from build123d import *

# Parameters (mm, degrees)
SKETCH2_R                    = 1.5875
MAINPLATE_DEPTH              = 8.89
SKETCH3_R                    = 3.4925
CASTERWHEEL_MOUNTHOLES_DEPTH = 3.048
SKETCH4_R                    = 2.159
ARDUINO_MOUNTHOLES_DEPTH     = 6.35
SKETCH5_R                    = 2.159
PDB_16A_MOUNTINGHOLES_DEPTH  = 6.35
SKETCH6_R                    = 2.232248555
PDB_15A_MOUNTINGHOLES_DEPTH  = 6.35
SKETCH7_R                    = 2.159
DRV8871_MOUNTINGHOLES_DEPTH  = 6.35
DRV8871_MOUNTPATTERN_COUNT   = 4
DRV8871_MOUNTPATTERN_PITCH   = 24.13
SKETCH8_R                    = 1.397
BOSS_EXTRUDE1_DEPTH          = 8.89
FILLET1_R                    = 2.54
FILLET2_R                    = 2.54


with BuildPart() as part:
    # Sketch2 → MainPlate (new body)
    with BuildSketch(Plane(origin=(0, 0, 0), x_dir=(1, 0, 0), z_dir=(0, 1, 0))):
        Polygon((-69.85, 0), (-69.85, 82.55), (69.85, 82.55), (69.85, 0), (69.85, -101.6), (-69.85, -101.6), align=None)
        with Locations(Location((30.1625, 19.05, 0), (0, 0, 270))):
            Circle(SKETCH2_R, mode=Mode.SUBTRACT)
        with Locations(Location((30.1625, -19.05, 0), (0, 0, 270))):
            Circle(SKETCH2_R, mode=Mode.SUBTRACT)
        with Locations(Location((-30.1625, -19.05, 0), (0, 0, 270))):
            Circle(SKETCH2_R, mode=Mode.SUBTRACT)
        with Locations(Location((-30.1625, 19.05, 0), (0, 0, 270))):
            Circle(SKETCH2_R, mode=Mode.SUBTRACT)
    extrude(amount=MAINPLATE_DEPTH)

    # Sketch3 → CasterWheel_MountHoles (cut)
    with BuildSketch(Plane(origin=(0, 8.89, 0), x_dir=(1, 0, 0), z_dir=(0, 1, 0))):
        with Locations(Location((-30.1625, 19.05, 0), (0, 0, 270))):
            Circle(SKETCH3_R)
        with Locations(Location((30.1625, 19.05, 0), (0, 0, 270))):
            Circle(SKETCH3_R)
        with Locations(Location((-30.1625, -19.05, 0), (0, 0, 270))):
            Circle(SKETCH3_R)
        with Locations(Location((30.1625, -19.05, 0), (0, 0, 270))):
            Circle(SKETCH3_R)
    extrude(amount=-CASTERWHEEL_MOUNTHOLES_DEPTH, mode=Mode.SUBTRACT)

    # Sketch4 → Arduino_MountHoles (cut)
    with BuildSketch(Plane(origin=(0, 8.89, 0), x_dir=(1, 0, 0), z_dir=(0, 1, 0))):
        with Locations(Location((-45.812177419, 59.587580645, 0), (0, 0, 270))):
            Circle(SKETCH4_R)
        with Locations(Location((-38.192177419, 11.327580645, 0), (0, 0, 270))):
            Circle(SKETCH4_R)
        with Locations(Location((36.737822581, 59.587580645, 0), (0, 0, 270))):
            Circle(SKETCH4_R)
        with Locations(Location((36.737822581, 11.327580645, 0), (0, 0, 270))):
            Circle(SKETCH4_R)
    extrude(amount=-ARDUINO_MOUNTHOLES_DEPTH, mode=Mode.SUBTRACT)

    # Sketch5 → PDB_16A_MountingHoles (cut)
    with BuildSketch(Plane(origin=(0, 8.89, 0), x_dir=(1, 0, 0), z_dir=(0, 1, 0))):
        with Locations(Location((-62.23, -5.588, 0), (0, 0, 270))):
            Circle(SKETCH5_R)
        with Locations(Location((-62.23, -95.25, 0), (0, 0, 270))):
            Circle(SKETCH5_R)
    extrude(amount=-PDB_16A_MOUNTINGHOLES_DEPTH, mode=Mode.SUBTRACT)

    # Sketch6 → PDB_15A_MountingHoles (cut)
    with BuildSketch(Plane(origin=(0, 8.89, 0), x_dir=(1, 0, 0), z_dir=(0, 1, 0))):
        with Locations(Location((-26.67, -95.25, 0), (0, 0, 270))):
            Circle(SKETCH6_R)
        with Locations(Location((-26.67, -12.192, 0), (0, 0, 270))):
            Circle(SKETCH6_R)
        with Locations(Location((11.43, -12.192, 0), (0, 0, 90))):
            Circle(SKETCH6_R)
        with Locations(Location((11.43, -95.25, 0), (0, 0, 90))):
            Circle(SKETCH6_R)
    extrude(amount=-PDB_15A_MOUNTINGHOLES_DEPTH, mode=Mode.SUBTRACT)

    # Sketch7 → DRV8871_MountingHoles (cut)
    with BuildSketch(Plane(origin=(0, 8.89, 0), x_dir=(1, 0, 0), z_dir=(0, 1, 0))):
        with Locations(Location((57.15, -97.155, 0), (0, 0, 270))):
            Circle(SKETCH7_R)
        with Locations(Location((57.15, -81.2165, 0), (0, 0, 270))):
            Circle(SKETCH7_R)
    drv8871_mountingholes = extrude(amount=-DRV8871_MOUNTINGHOLES_DEPTH, mode=Mode.SUBTRACT)

    # DRV8871_MountPattern: DRV8871_MountingHoles ×4
    with Locations(*[(0, 0, -i * DRV8871_MOUNTPATTERN_PITCH) for i in range(1, DRV8871_MOUNTPATTERN_COUNT)]):
        add(drv8871_mountingholes, mode=Mode.SUBTRACT)

    # Sketch8 → Boss-Extrude1 (add)
    with BuildSketch(Plane.XZ):
        Polygon((-69.85, 101.6), (-69.85, 66.675), (69.85, 66.675), (69.85, 101.6), (80.645, 101.6), (80.645, 93.98), (73.025, 93.98), (73.025, 67.31), (76.835, 67.31), (76.835, 59.69), (69.215, 59.69), (69.215, 63.5), (-69.215, 63.5), (-69.215, 59.69), (-76.835, 59.69), (-76.835, 67.31), (-73.025, 67.31), (-73.025, 93.98), (-80.645, 93.98), (-80.645, 101.6), align=None)
        with Locations(Location((-76.835, 97.79, 0), (0, 0, 270))):
            Circle(SKETCH8_R, mode=Mode.SUBTRACT)
        with Locations(Location((-73.025, 63.5, 0), (0, 0, 270))):
            Circle(SKETCH8_R, mode=Mode.SUBTRACT)
        with Locations(Location((73.025, 63.5, 0), (0, 0, 90))):
            Circle(SKETCH8_R, mode=Mode.SUBTRACT)
        with Locations(Location((76.835, 97.79, 0), (0, 0, 90))):
            Circle(SKETCH8_R, mode=Mode.SUBTRACT)
    extrude(amount=-BOSS_EXTRUDE1_DEPTH)

    # Fillet1
    fillet1_edges = [part.edges().sort_by_distance(p)[0] for p in [
        (-69.85, 4.445, 59.69),
        (69.85, 4.445, 59.69),
        (73.025, 4.445, 93.98),
        (73.025, 4.445, 67.31),
        (-73.025, 4.445, 67.31),
        (-73.025, 4.445, 93.98),
    ]]
    fillet(fillet1_edges, radius=FILLET1_R)

    # Fillet2
    fillet2_edges = [part.edges().sort_by_distance(p)[0] for p in [
        (-69.85, 4.445, -82.55),
        (-76.835, 4.445, 59.69),
        (-76.835, 4.445, 67.31),
        (-80.645, 4.445, 93.98),
        (-80.645, 4.445, 101.6),
        (69.85, 4.445, -82.55),
        (76.835, 4.445, 59.69),
        (76.835, 4.445, 67.31),
        (80.645, 4.445, 93.98),
        (80.645, 4.445, 101.6),
    ]]
    fillet(fillet2_edges, radius=FILLET2_R)


solid = part.part
Here's how the part is built. I have some questions about the finished solid (model axes, mm). A direction names the side the tool comes from. Give positions to 0.01 mm unless a question says otherwise; leave off trailing zeros. Order: outer loops, then holes, each group sorted by start corner. A loop starts at its lowest first (then second) coordinate and runs counter-clockwise, first axis right, second up. Notation, with made-up numbers: (45, -11.5) -> (62, -11.5) arc R27 ccw to (62, 6.5) -> close; hole circle Ø8 at (17.25, 29). An arc over 180 degrees is marked (long way). Use a Markdown table: item, result. Add a question column.
Item 1: Imagine slicing it at A-A on x = 11.43. Please give me the cut outline in (y, z), plus the area to 3 significant figures.
Item 2: For faces 1 (the face through (-27, 2.54, 95)), 2 (the face through (-73.025, 4, 80)), which set-ups out of +Z, -Z, +X, -X, +Y, -Y let a thin tool reach every point of the face, with its end or its side?
Item 3: Imagine slicing it at B-B on x = -62.23. Please give me the cut outline in (y, z).
Item 4: I need wall thicknesses on line 1 (X direction, y = 4.5, z = 19.05) (3 decimals); line 2 (Z direction, x = 37, y = 8); line 3 (Z direction, x = 11.43, y = 6). Which ranges of each line are inside material? Lowest first, please.
Item 5: Will these pins go through, and if not, where does the flat tip stop? pin 1 (2.5 mm diameter, centred on x = 57.15, z = 57.09, fed in from +Y); pin 2 (0.8 mm diameter, centred on x = -76.5, y = 3, fed in from -Z); pin 3 (6.5 mm diameter, centred on x = 30.16, z = -19.05, fed in from +Y); pin 4 (4.5 mm diameter, centred on x = 76.835, z = 97.79, fed in from +Y).
Item 6: Imagine slicing it at C-C on y = 4.25. Give the number of separate pieces and of enclosed holes in the cut face, plus the area to 3 significant figures.
Data:
| question | item | result |
|---|---|---|
| 1 | outline | (0, -82.55) -> (8.89, -82.55) -> (8.89, 9.96) -> (2.54, 9.96) -> (2.54, 14.42) -> (8.89, 14.42) -> (8.89, 93.02) -> (2.54, 93.02) -> (2.54, 97.48) -> (8.89, 97.48) -> (8.89, 101.6) -> (0, 101.6) -> close |
| 1 | area | 1,580 mm² |
| 2 | face 1 | +Y |
| 2 | face 2 | -X, +Y, -Y |
| 3 | outline | (0, -82.55) -> (8.89, -82.55) -> (8.89, 3.43) -> (2.54, 3.43) -> (2.54, 7.75) -> (8.89, 7.75) -> (8.89, 93.09) -> (2.54, 93.09) -> (2.54, 97.41) -> (8.89, 97.41) -> (8.89, 101.6) -> (0, 101.6) -> close |
| 4 | line 1 | x = -69.85 to -31.75, -28.575 to 28.575, 31.75 to 69.85 |
| 4 | line 2 | z = -82.55 to -61.73, -57.44 to -13.47, -9.18 to 101.6 |
| 4 | line 3 | z = -82.55 to 9.96, 14.42 to 93.02, 97.48 to 101.6 |
| 5 | pin 1 | stops at y = 2.54 |
| 5 | pin 2 | stops at z = 60.44 |
| 5 | pin 3 | stops at y = 5.84 |
| 5 | pin 4 | stops at y = 8.89 |
| 6 | separate pieces | 1 |
| 6 | enclosed holes | 26 |
| 6 | area | 25,800 mm² |
